from build123d import *

# Parameters (mm, degrees)
F1_DEPTH       = 30
F3_D           = 3
F3_CSINK_D     = 6
F3_CSINK_ANGLE = 90
F4_DEPTH       = 30.0010001
F5_T1_DEPTH    = 35
F5_T3_DEPTH    = 34.6192422485
F5_T5_DEPTH    = 34.6187341795
F6_R           = 1
F7_R           = 2


# Not quite as in the source:
# - a fillet or chamfer that OpenCascade refuses, or shapes differently, is made with other operations: its cross-section is extruded or revolved along the edge and cut away or added


with BuildPart() as f1:
    # F0 (on Front) → F1 (new body)
    with BuildSketch(Plane.XZ):
        with BuildLine():
            Line((-17.9, 6.5), (-17.9, 0))
            Line((-17.9, 0), (17.9, 0))
            Line((17.9, 0), (17.9, 6.5))
            Line((17.9, 6.5), (15.8, 6.5))
            Line((15.8, 6.5), (15.8, 5.8830036334))
            add(Edge.make_bspline(
                [(15.8, 3.048985269), (17.1972432804, 4.4659944512), (15.8, 5.8830036334)],
                knots=[2.53206789, 2.53206789, 2.53206789, 3.7511174172, 3.7511174172, 3.7511174172], degree=2, weights=[1, 0.8199201727, 1]))
            Line((15.8, 3.048985269), (15.8, 1.5))
            Line((15.8, 1.5), (8, 1.5))
            Line((8, 1.5), (-8, 1.5))
            Line((-8, 1.5), (-15.8, 1.5))
            Line((-15.8, 1.5), (-15.8, 3.0492304381))
            add(Edge.make_bspline(
                [(-16.4293519812, 4.4659944512), (-16.4293519812, 3.687532865), (-15.8, 3.0492304381)],
                knots=[0, 0, 0, 0.6094662657, 0.6094662657, 0.6094662657], degree=2, weights=[1, 0.953927057, 1]))
            add(Edge.make_bspline(
                [(-15.8, 5.8827584643), (-16.4293519812, 5.2444560374), (-16.4293519812, 4.4659944512)],
                knots=[5.6737190415, 5.6737190415, 5.6737190415, 6.2831853072, 6.2831853072, 6.2831853072], degree=2, weights=[1, 0.953927057, 1]))
            Line((-15.8, 5.8827584643), (-15.8, 6.5))
            Line((-15.8, 6.5), (-17.9, 6.5))
        make_face()
        with BuildLine():
            add(Edge.make_bspline(
                [(-15.8, 3.0492304381), (-9.4383519812, -3.4028909356), (-9.4383519812, 4.4659944512), (-9.4383519812, 12.334879838), (-15.8, 5.8827584643)],
                knots=[0.6094662657, 0.6094662657, 0.6094662657, 3.1415926536, 3.1415926536, 5.6737190415, 5.6737190415, 5.6737190415], degree=2, weights=[1, 0.3000386141, 1, 0.3000386141, 1]))
            Line((-15.8, 5.8827584643), (-15.8, 3.0492304381))
        make_face()
        with BuildLine():
            Line((-15.8, 3.0492304381), (-15.8, 5.8827584643))
            add(Edge.make_bspline(
                [(-15.8, 5.8827584643), (-16.4293519812, 5.2444560374), (-16.4293519812, 4.4659944512)],
                knots=[5.6737190415, 5.6737190415, 5.6737190415, 6.2831853072, 6.2831853072, 6.2831853072], degree=2, weights=[1, 0.953927057, 1]))
            add(Edge.make_bspline(
                [(-16.4293519812, 4.4659944512), (-16.4293519812, 3.687532865), (-15.8, 3.0492304381)],
                knots=[0, 0, 0, 0.6094662657, 0.6094662657, 0.6094662657], degree=2, weights=[1, 0.953927057, 1]))
        make_face()
        with BuildLine():
            add(Edge.make_bspline(
                [(15.8, 3.048985269), (17.1972432804, 4.4659944512), (15.8, 5.8830036334)],
                knots=[2.53206789, 2.53206789, 2.53206789, 3.7511174172, 3.7511174172, 3.7511174172], degree=2, weights=[1, 0.8199201727, 1]))
            Line((15.8, 5.8830036334), (15.8, 3.048985269))
        make_face()
        with BuildLine():
            Line((15.8, 3.048985269), (15.8, 5.8830036334))
            add(Edge.make_bspline(
                [(15.8, 5.8830036334), (9.4382216203, 12.3347779991), (9.4382216203, 4.4659944512)],
                knots=[3.7511174172, 3.7511174172, 3.7511174172, 6.2831853072, 6.2831853072, 6.2831853072], degree=2, weights=[1, 0.3000665154, 1]))
            add(Edge.make_bspline(
                [(9.4382216203, 4.4659944512), (9.4382216203, -3.4027890967), (15.8, 3.048985269)],
                knots=[0, 0, 0, 2.53206789, 2.53206789, 2.53206789], degree=2, weights=[1, 0.3000665154, 1]))
        make_face()
    extrude(amount=F1_DEPTH)

    # F3 (through all)
    with Locations(Plane.XY.offset(1.5)):
        with Locations((0, -15)):
            CounterSinkHole(F3_D / 2, F3_CSINK_D / 2, counter_sink_angle=F3_CSINK_ANGLE)

    # F0 (on Front) → F4 (cut, through all)
    with BuildSketch(Plane.XZ):
        with BuildLine():
            Line((15.8, 3.048985269), (15.8, 5.8830036334))
            add(Edge.make_bspline(
                [(15.8, 5.8830036334), (9.4382216203, 12.3347779991), (9.4382216203, 4.4659944512)],
                knots=[3.7511174172, 3.7511174172, 3.7511174172, 6.2831853072, 6.2831853072, 6.2831853072], degree=2, weights=[1, 0.3000665154, 1]))
            add(Edge.make_bspline(
                [(9.4382216203, 4.4659944512), (9.4382216203, -3.4027890967), (15.8, 3.048985269)],
                knots=[0, 0, 0, 2.53206789, 2.53206789, 2.53206789], degree=2, weights=[1, 0.3000665154, 1]))
        make_face()
        with BuildLine():
            add(Edge.make_bspline(
                [(15.8, 3.048985269), (17.1972432804, 4.4659944512), (15.8, 5.8830036334)],
                knots=[2.53206789, 2.53206789, 2.53206789, 3.7511174172, 3.7511174172, 3.7511174172], degree=2, weights=[1, 0.8199201727, 1]))
            Line((15.8, 5.8830036334), (15.8, 3.048985269))
        make_face()
        with BuildLine():
            add(Edge.make_bspline(
                [(-15.8, 3.0492304381), (-9.4383519812, -3.4028909356), (-9.4383519812, 4.4659944512), (-9.4383519812, 12.334879838), (-15.8, 5.8827584643)],
                knots=[0.6094662657, 0.6094662657, 0.6094662657, 3.1415926536, 3.1415926536, 5.6737190415, 5.6737190415, 5.6737190415], degree=2, weights=[1, 0.3000386141, 1, 0.3000386141, 1]))
            Line((-15.8, 5.8827584643), (-15.8, 3.0492304381))
        make_face()
        with BuildLine():
            Line((-15.8, 3.0492304381), (-15.8, 5.8827584643))
            add(Edge.make_bspline(
                [(-15.8, 5.8827584643), (-16.4293519812, 5.2444560374), (-16.4293519812, 4.4659944512)],
                knots=[5.6737190415, 5.6737190415, 5.6737190415, 6.2831853072, 6.2831853072, 6.2831853072], degree=2, weights=[1, 0.953927057, 1]))
            add(Edge.make_bspline(
                [(-16.4293519812, 4.4659944512), (-16.4293519812, 3.687532865), (-15.8, 3.0492304381)],
                knots=[0, 0, 0, 0.6094662657, 0.6094662657, 0.6094662657], degree=2, weights=[1, 0.953927057, 1]))
        make_face()
    extrude(amount=F4_DEPTH, mode=Mode.SUBTRACT)

    # F5: fillet of radius 1 on 4 edges, made by hand

    # F5_s2 → F5_t1 (cut)
    with BuildSketch(Plane.XZ.offset(-2.5)):
        with BuildLine():
            ThreePointArc((-17.9, 5.5), (-17.6071067812, 6.2071067812), (-16.9, 6.5))
            Line((-16.9, 6.5), (-17.9, 6.5))
            Line((-17.9, 6.5), (-17.9, 5.5))
        make_face()
        with BuildLine():
            ThreePointArc((16.9, 6.5), (17.6071067812, 6.2071067812), (17.9, 5.5))
            Line((17.9, 5.5), (17.9, 6.5))
            Line((17.9, 6.5), (16.9, 6.5))
        make_face()
    extrude(amount=F5_T1_DEPTH, mode=Mode.SUBTRACT)

    # F5_s4 → F5_t3 (cut)
    with BuildSketch(Plane.XZ.offset(-2.3096211243)):
        with BuildLine():
            ThreePointArc((-16.7238484497, 6.5), (-16.1683119812, 6.331492172), (-15.8, 5.8827584643))
            Line((-15.8, 5.8827584643), (-15.8, 6.5))
            Line((-15.8, 6.5), (-16.7238484497, 6.5))
        make_face()
    extrude(amount=F5_T3_DEPTH, mode=Mode.SUBTRACT)

    # F5_s6 → F5_t5 (cut)
    with BuildSketch(Plane.XZ.offset(-2.3093670897)):
        with BuildLine():
            ThreePointArc((15.8, 5.8830036334), (16.1683207082, 6.3315658823), (16.7237468359, 6.5))
            Line((16.7237468359, 6.5), (15.8, 6.5))
            Line((15.8, 6.5), (15.8, 5.8830036334))
        make_face()
    extrude(amount=F5_T5_DEPTH, mode=Mode.SUBTRACT)

    # F6
    f6_edges = [f1.edges().sort_by_distance(p)[0] for p in [
        (-15.8, -15, 1.5),
        (15.8, -15, 1.5),
    ]]
    fillet(f6_edges, radius=F6_R)

    # F7
    f7_edges = [f1.edges().sort_by_distance(p)[0] for p in [
        (-17.9, -15, 0),
        (17.9, -15, 0),
    ]]
    fillet(f7_edges, radius=F7_R)


solid = f1.part
Input: part model. Units: mm. Frame: model coordinates. A direction names the side the tool comes from. Give positions to 0.01 mm unless a question says otherwise; leave off trailing zeros. Order: outer loops, then holes, each group sorted by start corner. A loop starts at its lowest first (then second) coordinate and runs counter-clockwise, first axis right, second up. Notation, with made-up numbers: M -3.75,-26.75 L 6.25,-26.75 A20 cw 6.25,-16.75 Z; hole C 80,-14.5 d11. An arc over 180 degrees is marked long. Answer as a JSON object with one key per item and string values.
1. Cut plane B-B, the plane z = 1. Output: boundary loops of the cut face in (x, y), and give its area (3 significant figures).
Result sheet:
{"outline": "M -17.63,-30 L 17.63,-30 L 17.63,0 L -17.63,0 Z; hole C 0,-15 d5", "area": "1,040 mm²"}
2. Reachability of faces 5 (the cylindrical face through (-17.33, -15.21, 0.6)), 6 (the cylindrical face through (-16.18, -14.79, 6.34)) from +Z, -Z, +X, -X, +Y, -Y: full face, straight path, thin tool, end or side. Return the list, or none.
Result sheet:
{"face 5": "-Z, -X, +Y, -Y", "face 6": "+Z, +Y, -Y"}
3. Pull-direction query (X, two-part tool) for faces 1 (the flat face through (0, -11, 0)), 2 (the cylindrical face through (16.161, -14.79, 6.327)), 3 (the flat face through (-17.9, -15, 4)), 4 (the cylindrical face through (17.3, -15.21, 0.57)); classes: +X half, -X half, draft (parallel to the pull), parting line (faces both ways), or undercut.
Result sheet:
{"face 1": "draft", "face 2": "undercut", "face 3": "-X half", "face 4": "+X half"}
4. First-contact query: P1, Ø8, axis at x = 5.5, y = -25, coming from the +Z side. Flat tip, straight axial feed; report the tip coordinate or a pass-through.
Result sheet:
{"P1": "z = 1.5"}
5. Cut plane A-A, the plane x = 0. Output: boundary loops of the cut face in (y, z).
Result sheet:
{"outline": "M -30,0 L -16.5,0 L -18,1.5 L -30,1.5 Z; M -13.5,0 L 0,0 L 0,1.5 L -12,1.5 Z"}
6. Ray query, line 1 (X direction, y = -19.5, z = 4.5); line 2 (Z direction, x = 4, y = -18); line 3 (X direction, y = -27, z = 3.75). Return the intervals inside material, ascending. Write a range as [from, to].
Result sheet:
{"line 1": "[-17.9, -16.43], [16.43, 17.9]", "line 2": "[0, 1.5]", "line 3": "[-17.9, -16.28], [16.28, 17.9]"}
